Could you check a few things on this drawing? It's one solid part, dimensions in mm from its lowest x, y, z. Round coordinates to 2 decimals unless told otherwise and drop trailing zeros. Loops run counter-clockwise (first coordinate to the right, second up) from the corner with the lowest first, then second, coordinate; pieces in that order, holes last. Notation, with made-up numbers: M -12,21.5 L 22,21.5 A9 ccw 22,32.5 Z; hole C 11.5,73 d2. An arc over 180 degrees is marked long. Return JSON: item names as keys, results as strings.
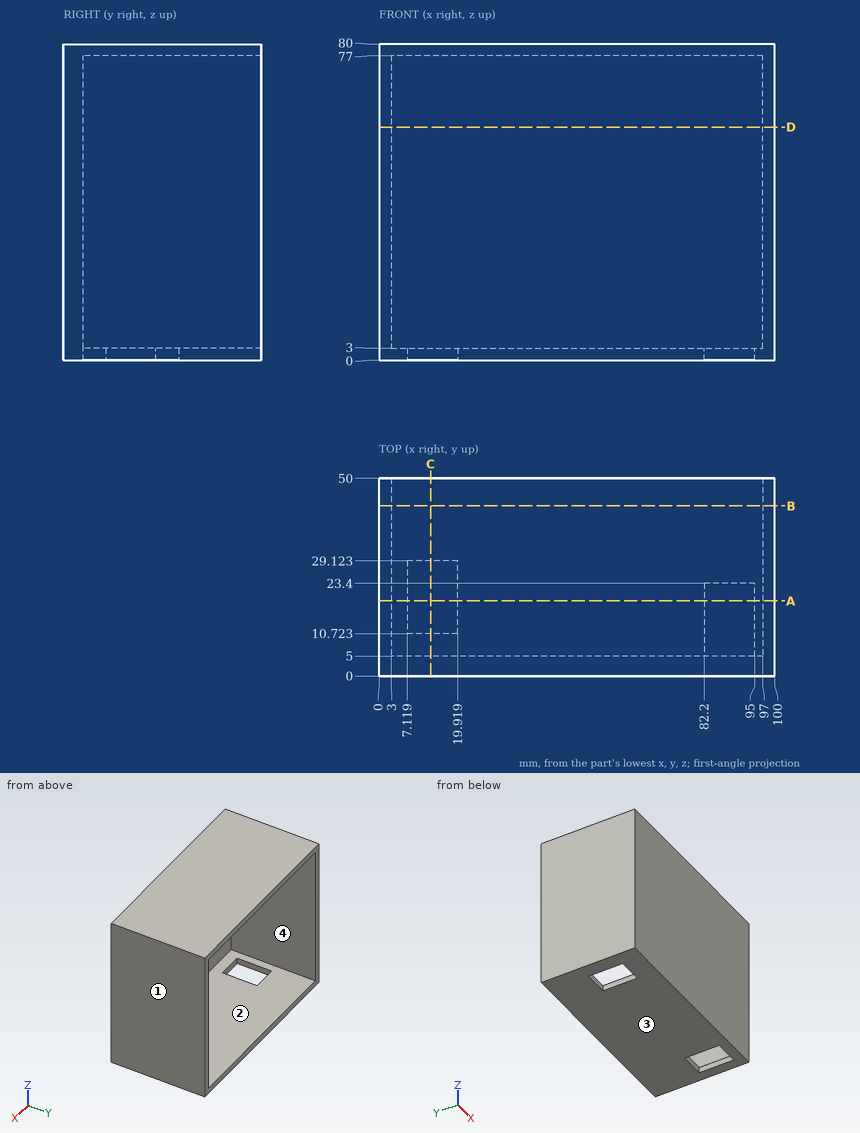
Q1. Thinking about a two-plate mould opening in Z: for the marked faces 1, 2, 3 and 4, which applies, pulls with the +Z half, pulls with the -Z half, needs draft (parallel to the pull), parting line crosses it, or undercut?
Results:
{"face 1": "needs draft", "face 2": "undercut", "face 3": "pulls with the -Z half", "face 4": "undercut"}
Q2. I'm going to push a flat-ended pin straight in: pin 1 Ø4 at (x, z) = (48.5, 46.5) entering from +Y. Where does the tip first touch, or does it pass through?
Results:
{"pin 1": "stops at y = 5"}
Q3. If I drill on line 1 along Z through (x, y) = (72.5, 44); line 2 along X through (y, z) = (6, 35.5); line 3 along Y through (x, z) = (83.5, 28.5), over which ranges is the centre line in solid material (lowest first)?
Results:
{"line 1": "z = 0 to 3, 77 to 80", "line 2": "x = 0 to 3, 97 to 100", "line 3": "y = 0 to 5"}
Q4. Suppose I cut it at C-C, the plane x = 13. Please give me the cut outline in (y, z).
Results:
{"outline": "M 0,0 L 10.72,0 L 10.72,3 L 5,3 L 5,77 L 50,77 L 50,80 L 0,80 Z; M 29.12,0 L 50,0 L 50,3 L 29.12,3 Z"}
Q5. Suppose I cut it at D-D, the plane z = 59. Please give me the cut outline in (x, y).
Results:
{"outline": "M 0,0 L 100,0 L 100,50 L 97,50 L 97,5 L 3,5 L 3,50 L 0,50 Z"}
Q6. Suppose I cut it at B-B, the plane y = 43. Please give me the cut outline in (x, z), plus the area to 3 significant figures.
Results:
{"outline": "M 0,0 L 100,0 L 100,80 L 0,80 Z; hole M 3,3 L 97,3 L 97,77 L 3,77 Z", "area": "1,040 mm2"}
Q7. Suppose I cut it at A-A, the plane y = 19. Please give me the cut outline in (x, z).
Results:
{"outline": "M 0,0 L 7.12,0 L 7.12,3 L 3,3 L 3,77 L 97,77 L 97,3 L 95,3 L 95,0 L 100,0 L 100,80 L 0,80 Z; M 19.92,0 L 82.2,0 L 82.2,3 L 19.92,3 Z"}
